from build123d import *

# Parameters (mm, degrees)
SKETCH1_W           = 20
SKETCH1_H           = 12
SKETCH1_R           = 3.15
SKETCH1_W_2         = 85
SKETCH1_H_2         = 3
BOSS_EXTRUDE1_DEPTH = 230
SKETCH2_W           = 200
SKETCH2_H           = 15
CUT_EXTRUDE1_DEPTH  = 210
SKETCH3_W           = 43.6
SKETCH3_H           = 137.6
SKETCH3_W_2         = 37
SKETCH3_H_2         = 131
BOSS_EXTRUDE2_DEPTH = 12
CUT_EXTRUDE2_DEPTH  = 199.566588327
SKETCH6_R           = 2.5
CUT_EXTRUDE3_DEPTH  = 150
SKETCH7_W           = 25
SKETCH7_H           = 40
CUT_EXTRUDE4_DEPTH  = 150


with BuildPart() as part:
    # Sketch1 → Boss-Extrude1 (new body)
    # profile 1 of 3: a face of its own
    with BuildSketch(Plane.XY):
        with Locations((-25, -1)):
            Rectangle(SKETCH1_W, SKETCH1_H)
        with Locations((-25, 0)):
            Circle(SKETCH1_R, mode=Mode.SUBTRACT)
    # profile 2 of 3: a face of its own
    with BuildSketch(Plane.XY):
        with Locations((25, -1)):
            Rectangle(SKETCH1_W, SKETCH1_H)
        with Locations((25, 0)):
            Circle(SKETCH1_R, mode=Mode.SUBTRACT)
    # profile 3 of 3: a face of its own
    with BuildSketch(Plane.XY):
        with Locations((0, 6.5)):
            Rectangle(SKETCH1_W_2, SKETCH1_H_2)
    extrude(amount=BOSS_EXTRUDE1_DEPTH)

    # Sketch2 → Cut-Extrude1 (cut)
    with BuildSketch(Plane.ZY.offset(35)):
        with Locations((115, -2.5)):
            Rectangle(SKETCH2_W, SKETCH2_H)
    extrude(amount=-CUT_EXTRUDE1_DEPTH, mode=Mode.SUBTRACT)

    # Sketch3 → Boss-Extrude2 (add)
    with BuildSketch(Plane.XZ.offset(-5)):
        with Locations((0, 105)):
            Rectangle(SKETCH3_W, SKETCH3_H)
        with Locations((0, 105)):
            Rectangle(SKETCH3_W_2, SKETCH3_H_2, mode=Mode.SUBTRACT)
    extrude(amount=BOSS_EXTRUDE2_DEPTH)

    # Sketch4 → Cut-Extrude2 (cut, through all)
    with BuildSketch(Plane(origin=(0, 0, 36.2), x_dir=(-1, 0, 0), z_dir=(0, 0, -1))):
        Polygon((0, 0), (-7.5, 0), (-7.5, -8), (7.5, -8), (7.5, 0), align=None)
    extrude(amount=-CUT_EXTRUDE2_DEPTH, mode=Mode.SUBTRACT)

    # Sketch6 → Cut-Extrude3 (cut)
    with BuildSketch(Plane(origin=(0, 0, 36.2), x_dir=(-1, 0, 0), z_dir=(0, 0, -1))):
        with Locations((-12, -4)):
            Circle(SKETCH6_R)
        with Locations((12, -4)):
            Circle(SKETCH6_R)
    extrude(amount=-CUT_EXTRUDE3_DEPTH, mode=Mode.SUBTRACT)

    # Sketch7 → Cut-Extrude4 (cut)
    with BuildSketch(Plane(origin=(0, 8, 0), x_dir=(1, 0, 0), z_dir=(0, 1, 0))):
        Rectangle(SKETCH7_W, SKETCH7_H)
    extrude(amount=-CUT_EXTRUDE4_DEPTH, mode=Mode.SUBTRACT)


solid = part.part
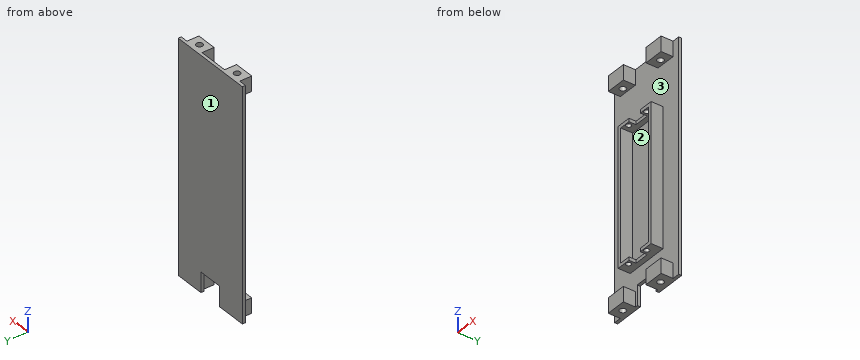
Build history of the part. All positions in model axes, mm. Face numbers are marked on the shaded views. Coordinates: 2 decimals unless noted, no trailing zeros. Order: outer loops, then holes, each group sorted by start corner. A loop starts at its lowest first (then second) coordinate and runs counter-clockwise, first axis right, second up. Notation, with made-up numbers: (-28, -6) - (16, -6) arc R27 ccw to (16, 32) - close; hole circle Ø1 at (-32, -38). An arc over 180 degrees is marked (long way). Write each question's results on one line, items separated by ' | '. Start each with the question number.
Item 1: Band-saw the part on D-D on z = 201.5. Write the cut outline in (x, y), and give its area (3 significant figures).
Item 2: Wall check: probe 1 along X at (y, z) = (0, 3); probe 2 along Y at (x, z) = (25, 4); probe 3 along Z at (x, y) = (-32, -5.5). Give the ranges that are in metal, low to high. Write a range as [from, to].
Item 3: Flat gauge pins, fed straight in: pin 1 (8 mm diameter, centred on x = 25, y = 0, fed in from +Z); pin 2 (3.5 mm diameter, centred on y = 0, z = 222, fed in from -X); pin 3 (1 mm diameter, centred on x = -1.5, z = 172, fed in from -Y); pin 4 (5 mm diameter, centred on y = -1.5, z = 74.5, fed in from -X). Where does each tip first touch, or does it go through?
Item 4: Mould opens along Z. For the marked faces 1, 2 and 3 say: released by +Z, released by -Z, zero draft, split by the parting line, or undercut.
Item 5: Band-saw the part on B-B on z = 47. Write the cut outline in (x, y).
Item 6: Band-saw the part on A-A on x = 25. Write the cut outline in (y, z), and give its area (3 significant figures).
Item 7: Band-saw the part on C-C on x = -0.5. Write the cut outline in (y, z).
Numbers:
1) outline: (-42.5, 5) - (42.5, 5) - (42.5, 8) - (-42.5, 8) - close | area: 255 mm^2
2) probe 1: [-35, -28.15], [-21.85, -15], [15, 21.85], [28.15, 35] | probe 2: [-7, -3.15], [3.15, 8] | probe 3: [0, 15], [215, 230]
3) pin 1: z = 230 | pin 2: x = -35 | pin 3: y = 0 | pin 4: x = -21.8
4) face 1: zero draft | face 2: undercut | face 3: undercut
5) outline: (-42.5, 5) - (-21.8, 5) - (-21.8, -7) - (-18.5, -7) - (-18.5, 5) - (18.5, 5) - (18.5, -7) - (21.8, -7) - (21.8, 5) - (42.5, 5) - (42.5, 8) - (-42.5, 8) - close
6) outline: (-7, 0) - (-3.15, 0) - (-3.15, 15) - (-7, 15) - close; (-7, 215) - (-3.15, 215) - (-3.15, 230) - (-7, 230) - close; (3.15, 0) - (8, 0) - (8, 230) - (3.15, 230) - (3.15, 215) - (5, 215) - (5, 15) - (3.15, 15) - close | area: 861 mm^2
7) outline: (0, 36.2) - (5, 36.2) - (5, 20) - (8, 20) - (8, 230) - (5, 230) - (5, 173.8) - (0, 173.8) - (0, 170.5) - (5, 170.5) - (5, 39.5) - (0, 39.5) - close
